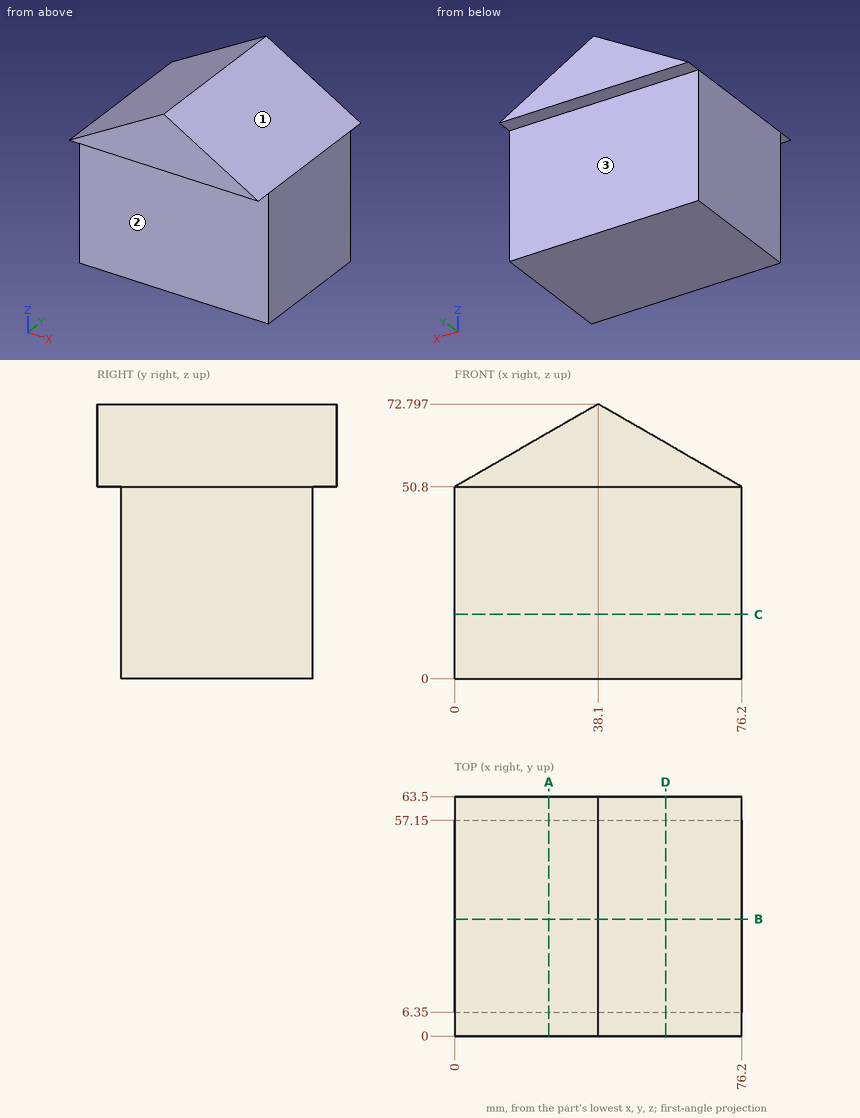
Verification items for this drawing (mm, ordinates from the low corner). A direction names the side the tool comes from. Round coordinates to 2 decimals unless told otherwise and drop trailing zeros. Write each loop counter-clockwise with the first axis right and the second up, starting at its lowest first coordinate (ties: lowest second). Pieces come first, ordered by that corner, then holes. Notation, with made-up numbers: (35.25, -28) - (89.25, -28) arc R12 ccw to (89.25, -18) - close; hole circle Ø3 at (20, -16.75). An arc over 180 degrees is marked (long way). One line per item, written item: value.
1. Scan lines: L1, parallel to Y at x = 14.5, z = 40; L2, parallel to X at y = 61.5, z = 68.5; L3, parallel to Z at x = 34, y = 39. Record each from-to range of solid material in increasing order.
The answers:
L1: y = 6.35 to 57.15
L2: x = 30.66 to 45.54
L3: z = 0 to 70.43
2. Cross-section at C-C on z = 17. Record the boundary of the cut face in (x, y).
The answers:
outline: (0, 6.35) - (76.2, 6.35) - (76.2, 57.15) - (0, 57.15) - close
3. Cross-section at B-B on y = 31. Record the boundary of the cut face in (x, z), and give its area (3 significant figures).
The answers:
outline: (0, 0) - (76.2, 0) - (76.2, 50.8) - (38.1, 72.8) - (0, 50.8) - close
area: 4,710 mm^2
4. Depth check by flat-ended pin: pin 1 Ø1.9 at (x, y) = (31.5, 60.5) entering from -Z; pin 2 Ø4 at (x, y) = (20, 22) entering from +Z; pin 3 Ø4 at (x, z) = (20.5, 18) entering from -Y; pin 4 Ø6 at (y, z) = (19.5, 19) entering from -X. Enter the tip coordinate at first touch or a pass-through.
The answers:
pin 1: stops at z = 50.8
pin 2: stops at z = 63.5
pin 3: stops at y = 6.35
pin 4: stops at x = 0
5. Cross-section at A-A on x = 25. Record the boundary of the cut face in (y, z).
The answers:
outline: (0, 50.8) - (6.35, 50.8) - (6.35, 0) - (57.15, 0) - (57.15, 50.8) - (63.5, 50.8) - (63.5, 65.23) - (0, 65.23) - close
6. Cross-section at D-D on x = 56. Record the boundary of the cut face in (y, z).
The answers:
outline: (0, 50.8) - (6.35, 50.8) - (6.35, 0) - (57.15, 0) - (57.15, 50.8) - (63.5, 50.8) - (63.5, 62.46) - (0, 62.46) - close
7. Set-up check for the marked faces 1, 2 and 3: record each of +Z, -Z, +X, -X, +Y, -Y from which the full face is reachable in a straight line by a thin tool's end or side.
The answers:
face 1: +Z, +X, +Y, -Y
face 2: -Z, +X, -X, -Y
face 3: -Z, +X, -X, +Y
